from build123d import *

# Parameters (mm, degrees)
BOSS_EXTRUDE1_DEPTH = 6
SHELL1_T            = -2
SKETCH3_R           = 2
CUT_EXTRUDE1_DEPTH  = 32.894356868
SKETCH9_R           = 1.5
CUT_EXTRUDE6_DEPTH  = 32.894356868
SKETCH11_R          = 2
CUT_EXTRUDE7_DEPTH  = 32.579265349
SKETCH12_W          = 6.5
SKETCH12_H          = 8
CUT_EXTRUDE8_DEPTH  = 1
SKETCH13_R          = 0.6
CUT_EXTRUDE9_DEPTH  = 0.5


with BuildPart() as part:
    # Sketch1 → Boss-Extrude1 (new body)
    with BuildSketch(Plane.XY):
        Polygon((17, -7), (-27.5, -7), (-27.5, 7), (27.5, 7), (27.5, -7), (27.5, -15), (17, -15), align=None)
    extrude(amount=BOSS_EXTRUDE1_DEPTH)

    # Shell1
    shell1_openings = [part.faces().sort_by_distance(p)[0] for p in [
        (2.18852459, -1.081967213, 6),
    ]]
    offset(amount=SHELL1_T, openings=shell1_openings, kind=Kind.INTERSECTION)

    # Sketch3 → Cut-Extrude1 (cut, through all)
    with BuildSketch(Plane(origin=(0, 0, 0), x_dir=(-1, 0, 0), z_dir=(0, 0, -1))):
        with Locations((-21, -1.5)):
            Circle(SKETCH3_R)
        with Locations((-14.45, -1.5)):
            Circle(SKETCH3_R)
        with Locations((-7.9, -1.5)):
            Circle(SKETCH3_R)
        with Locations((-1.35, -1.5)):
            Circle(SKETCH3_R)
        with Locations((5.2, -1.5)):
            Circle(SKETCH3_R)
        with Locations((11.75, -1.5)):
            Circle(SKETCH3_R)
        with Locations((18.3, -1.5)):
            Circle(SKETCH3_R)
    extrude(amount=-CUT_EXTRUDE1_DEPTH, mode=Mode.SUBTRACT)

    # Sketch9 → Cut-Extrude6 (cut, through all)
    with BuildSketch(Plane(origin=(0, 0, 0), x_dir=(-1, 0, 0), z_dir=(0, 0, -1))):
        with Locations((-17.5, 2.8)):
            Circle(SKETCH9_R)
        with Locations((8.5, 2.8)):
            Circle(SKETCH9_R)
    extrude(amount=-CUT_EXTRUDE6_DEPTH, mode=Mode.SUBTRACT)

    # Sketch11 → Cut-Extrude7 (cut, through all)
    with BuildSketch(Plane.XY.offset(2)):
        with Locations((22.25, -10)):
            Circle(SKETCH11_R)
    extrude(amount=-CUT_EXTRUDE7_DEPTH, mode=Mode.SUBTRACT)

    # Sketch12 → Cut-Extrude8 (cut)
    with BuildSketch(Plane.XY.offset(2)):
        with Locations((22.25, -9)):
            Rectangle(SKETCH12_W, SKETCH12_H)
    extrude(amount=-CUT_EXTRUDE8_DEPTH, mode=Mode.SUBTRACT)

    # Sketch13 → Cut-Extrude9 (cut)
    with BuildSketch(Plane.XY.offset(1)):
        with Locations((20.25, -8)):
            Circle(SKETCH13_R)
        with Locations((24.25, -8)):
            Circle(SKETCH13_R)
        with Locations((24.25, -12)):
            Circle(SKETCH13_R)
        with Locations((20.25, -12)):
            Circle(SKETCH13_R)
    extrude(amount=-CUT_EXTRUDE9_DEPTH, mode=Mode.SUBTRACT)


solid = part.part
Geometry check sheet. Reference: the model listing, model coordinates, mm. A direction names the side the tool comes from. Give positions to 0.01 mm unless a question says otherwise; leave off trailing zeros. Order: outer loops, then holes, each group sorted by start corner. A loop starts at its lowest first (then second) coordinate and runs counter-clockwise, first axis right, second up. Notation, with made-up numbers: (-29, 43) - (17, 43) arc R18 cw to (17, 61) - close; hole circle Ø9 at (26.25, -29.5). An arc over 180 degrees is marked (long way). Use one line per item in the form item = value.
1) Sectioned sample at B-B (z = 5.2). Record the boundary of the cut face in (x, y), and give its area (3 significant figures).
Working result:
outline = (-27.5, -7) - (17, -7) - (17, -15) - (27.5, -15) - (27.5, 7) - (-27.5, 7) - close; hole (-25.5, -5) - (19, -5) - (19, -13) - (25.5, -13) - (25.5, 5) - (-25.5, 5) - close
area = 292 mm^2
2) Sectioned sample at C-C (y = -1.5). Count the separate pieces of the cut face and the enclosed holes in it, and give its area (3 significant figures).
Working result:
separate_pieces = 8
enclosed_holes = 0
area = 70.0 mm^2
3) Draft check along X on faces 1 (the face through (4, -6, 6)), 2 (the face through (-3, -5, 4)), 3 (the face through (27.5, -4, 3)), 4 (the face through (-16.302, -1.412, 0.986)). Enter one of: released by +X, released by -X, zero draft, split by the parting line, or undercut.
Working result:
face_1 = zero draft
face_2 = undercut
face_3 = released by +X
face_4 = undercut
4) Material ranges on probe 1 along X at (y, z) = (-2.25, 5); probe 2 along Y at (x, z) = (-11.75, 0.55); probe 3 along X at (y, z) = (-12.5, 5.65), recorded low to high. Write a range as from..to.
Working result:
probe_1 = -27.5..-25.5, 25.5..27.5
probe_2 = -7..-3.5, 0.5..7
probe_3 = 17..19, 25.5..27.5
5) Access from +Z, -Z, +X, -X, +Y, -Y to the whole of each face (thin tool, end or side, straight path). Record for faces 5 (the face through (22.2, -5, 1.5)), 6 (the face through (3.348, -1.412, 0.986)).
Working result:
face_5 = +Z
face_6 = +Z, -Z
6) Depth check by flat-ended pin: pin 1 Ø3 at (x, y) = (21, -1.5) entering from -Z; pin 2 Ø3 at (x, z) = (1.5, 2) entering from -Y; pin 3 Ø2 at (y, z) = (-10, 3.5) entering from -X; pin 4 Ø3 at (x, y) = (18, -1.5) entering from +Z. Enter the tip coordinate at first touch or a pass-through.
Working result:
pin_1 = through
pin_2 = -7
pin_3 = 17
pin_4 = 2
7) Sectioned sample at D-D (x = -11.75). Record the boundary of the cut face in (y, z), and give its area (3 significant figures).
Working result:
outline = (-7, 0) - (-3.5, 0) - (-3.5, 2) - (-5, 2) - (-5, 6) - (-7, 6) - close; (0.5, 0) - (7, 0) - (7, 6) - (5, 6) - (5, 2) - (0.5, 2) - close
area = 36.0 mm^2
8) Sectioned sample at A-A (x = 17.5). Record the boundary of the cut face in (y, z), and give its area (3 significant figures).
Working result:
outline = (-15, 0) - (1.3, 0) - (1.3, 2) - (-5, 2) - (-5, 6) - (-15, 6) - close; (4.3, 0) - (7, 0) - (7, 6) - (5, 6) - (5, 2) - (4.3, 2) - close
area = 86.0 mm^2
